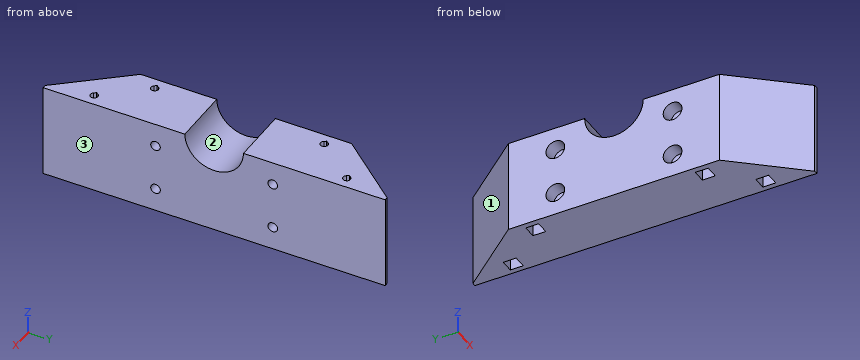
```python
from build123d import *

# Parameters (mm, degrees)
BOSS_EXTRUDE1_DEPTH   = 40
SKETCH2_R             = 2.05
CUT_EXTRUDE1_DEPTH    = 25.8
SKETCH2_4_R           = 4
SKETCH2_4_R_2         = 2.05
CUT_EXTRUDE2_DEPTH    = 6
CHAMFER1_SIZE2        = 2.5
CHAMFER1_SIZE         = 1.775056745
CHAMFER1_EDGE_2_SIZE2 = 2.5
CHAMFER1_EDGE_2_SIZE  = 1.775056745
SKETCH3_W             = 5.5
SKETCH3_H             = 5.5
CUT_EXTRUDE3_DEPTH    = 5


with BuildPart() as part:
    # Sketch1 → Boss-Extrude1 (new body)
    with BuildSketch(Plane(origin=(0, 0, 0), x_dir=(0, 1, 0), z_dir=(0, 0, 1))):
        Polygon((-45, 25), (45, 25), (74.76, 0.2), (-74.76, 0.2), align=None)
        with BuildLine():
            Line((-54.771952061, 6.432118468), (-53.854229763, 7.074714539))
            Line((-53.854229763, 7.074714539), (-52.936507465, 6.432118468))
            ThreePointArc((-52.936507465, 6.432118468), (-53.854229763, 3.521475197), (-54.771952061, 6.432118468))
        make_face(mode=Mode.SUBTRACT)
        with BuildLine():
            Line((-37.063492535, 21.189168074), (-36.145770237, 21.831764145))
            Line((-36.145770237, 21.831764145), (-35.228047939, 21.189168074))
            ThreePointArc((-35.228047939, 21.189168074), (-36.145770237, 18.278524803), (-37.063492535, 21.189168074))
        make_face(mode=Mode.SUBTRACT)
        with BuildLine():
            Line((35.228047939, 21.189168074), (36.145770237, 21.831764145))
            Line((36.145770237, 21.831764145), (37.063492535, 21.189168074))
            ThreePointArc((37.063492535, 21.189168074), (36.145770237, 18.278524803), (35.228047939, 21.189168074))
        make_face(mode=Mode.SUBTRACT)
        with BuildLine():
            Line((52.936507465, 6.432118468), (53.854229763, 7.074714539))
            Line((53.854229763, 7.074714539), (54.771952061, 6.432118468))
            ThreePointArc((54.771952061, 6.432118468), (53.854229763, 3.521475197), (52.936507465, 6.432118468))
        make_face(mode=Mode.SUBTRACT)
    extrude(amount=-BOSS_EXTRUDE1_DEPTH)

    # Sketch2 → Cut-Extrude1 (cut, through all)
    with BuildSketch(Plane(origin=(-25, 0, 0), x_dir=(0, -1, 0), z_dir=(-1, 0, 0))):
        with Locations((-25, -10)):
            Circle(SKETCH2_R)
        with Locations((-25, -30)):
            Circle(SKETCH2_R)
        with Locations((25, -30)):
            Circle(SKETCH2_R)
        with Locations((25, -10)):
            Circle(SKETCH2_R)
        with BuildLine():
            Line((12.5, 0), (-12.5, 0))
            ThreePointArc((-12.5, 0), (0, -12.5), (12.5, 0))
        make_face()
    extrude(amount=-CUT_EXTRUDE1_DEPTH, mode=Mode.SUBTRACT)

    # Sketch2_4 → Cut-Extrude2 (cut)
    with BuildSketch(Plane(origin=(-25, 0, 0), x_dir=(0, -1, 0), z_dir=(-1, 0, 0))):
        with Locations((-25, -10)):
            Circle(SKETCH2_4_R)
        with Locations((-25, -10)):
            Circle(SKETCH2_4_R_2, mode=Mode.SUBTRACT)
        with Locations((-25, -30)):
            Circle(SKETCH2_4_R)
        with Locations((-25, -30)):
            Circle(SKETCH2_4_R_2, mode=Mode.SUBTRACT)
        with Locations((25, -10)):
            Circle(SKETCH2_4_R)
        with Locations((25, -10)):
            Circle(SKETCH2_4_R_2, mode=Mode.SUBTRACT)
        with Locations((25, -30)):
            Circle(SKETCH2_4_R)
        with Locations((25, -30)):
            Circle(SKETCH2_4_R_2, mode=Mode.SUBTRACT)
        with BuildLine():
            Line((-12.5, 0), (12.5, 0))
            ThreePointArc((12.5, 0), (0, -12.5), (-12.5, 0))
        make_face()
    extrude(amount=-CUT_EXTRUDE2_DEPTH, mode=Mode.SUBTRACT)

    # Chamfer1
    chamfer1_edges = [part.edges().sort_by_distance(p)[0] for p in [
        (-0.2, 74.76, -20),
    ]]
    chamfer(chamfer1_edges, length=CHAMFER1_SIZE, length2=CHAMFER1_SIZE2)

    # Chamfer1 edge 2
    chamfer1_edge_2_edges = [part.edges().sort_by_distance(p)[0] for p in [
        (-0.2, -74.76, -20),
    ]]
    chamfer(chamfer1_edge_2_edges, length=CHAMFER1_EDGE_2_SIZE, length2=CHAMFER1_EDGE_2_SIZE2)

    # Sketch3 → Cut-Extrude3 (cut)
    with BuildSketch(Plane(origin=(0, 0, -40), x_dir=(1, 0, 0), z_dir=(0, 0, -1))):
        with Locations((-19.878524803, 36.145770237)):
            Rectangle(SKETCH3_W, SKETCH3_H)
        with Locations((-5.121475197, 53.854229763)):
            Rectangle(SKETCH3_W, SKETCH3_H)
        with Locations((-19.878524803, -36.145770237)):
            Rectangle(SKETCH3_W, SKETCH3_H)
        with Locations((-5.121475197, -53.854229763)):
            Rectangle(SKETCH3_W, SKETCH3_H)
    extrude(amount=-CUT_EXTRUDE3_DEPTH, mode=Mode.SUBTRACT)


solid = part.part
```
Can you work these out from the model? Positions are in its coordinate system, mm. Face numbers are marked on the shaded views. Give positions to 0.01 mm unless a question says otherwise; leave off trailing zeros. Write each loop counter-clockwise with the first axis right and the second up, starting at its lowest first coordinate (ties: lowest second). Pieces come first, ordered by that corner, then holes. Notation, with made-up numbers: (-25, 65) - (-13, 65) arc R13 ccw to (-13, 86) - close; hole circle Ø8 at (9.25, 54.5). An arc over 180 degrees is marked (long way). Write item = value, one per line. Start each with the question number.
1. For pin 1 (3 mm diameter, centred on x = -19.88, y = 36.15, fed in from +Z); pin 2 (2.5 mm diameter, centred on y = -52.5, z = -38, fed in from -X); pin 3 (5 mm diameter, centred on x = -18, z = -33, fed in from -Y); pin 4 (6.5 mm diameter, centred on y = 25, z = -10, fed in from -X), each with a flat end and sliding along its axis, tell me the tip position at first contact or that it passes through.
2. Please list where these lines run through material, in increasing order: line 1 (Z direction, x = -20.85, y = 25); line 2 (Y direction, x = -7, z = -11); line 3 (Y direction, x = -19.75, z = -25.5).
3. Imagine slicing it at B-B (z = -23.5). Please give me the cut outline in (x, y).
4. Thinking about a two-plate mould opening in Y: for the marked faces 1, 2 and 3, which applies, released by +Y, released by -Y, zero draft, split by the parting line, or undercut?
5. Imagine slicing it at C-C (y = -25). Please give me the cut outline in (x, z), and give its area (3 significant figures).
6. Imagine slicing it at A-A (z = -30). Count the separate pieces of the cut face and the enclosed holes in it, and give its area (3 significant figures).
7. Imagine slicing it at D-D (x = -10.75). Please give me the cut outline in (y, z).
Worked answers:
q1.pin_1 = through
q1.pin_2 = -19.79
q1.pin_3 = -56.4
q1.pin_4 = -19
q2.line_1 = -40 to -34, -26 to -14, -6 to 0
q2.line_2 = -66.6 to -53.96, -53.75 to -26.79, -23.21 to -5.94, 5.94 to 23.21, 26.79 to 53.75, 53.96 to 66.6
q2.line_3 = -51.3 to -37.74, -34.55 to 34.55, 37.74 to 51.3
q3.outline = (-25, -45) - (-1.8, -72.84) - (-0.2, -72.98) - (-0.2, 72.98) - (-1.8, 72.84) - (-25, 45) - close; hole (-21.83, -36.15) - (-21.19, -37.06) arc R1.6 ccw (long way) to (-21.19, -35.23) - close; hole (-21.83, 36.15) - (-21.19, 35.23) arc R1.6 ccw (long way) to (-21.19, 37.06) - close; hole (-7.07, -53.85) - (-6.43, -54.77) arc R1.6 ccw (long way) to (-6.43, -52.94) - close; hole (-7.07, 53.85) - (-6.43, 52.94) arc R1.6 ccw (long way) to (-6.43, 54.77) - close
q4.face_1 = released by +Y
q4.face_2 = undercut
q4.face_3 = zero draft
q5.outline = (-25, -40) - (-0.2, -40) - (-0.2, -32.05) - (-19, -32.05) - (-19, -34) - (-25, -34) - close; (-25, -26) - (-19, -26) - (-19, -27.95) - (-0.2, -27.95) - (-0.2, -12.05) - (-19, -12.05) - (-19, -14) - (-25, -14) - close; (-25, -6) - (-19, -6) - (-19, -7.95) - (-0.2, -7.95) - (-0.2, 0) - (-25, 0) - close
q5.area = 742 mm2
q6.separate_pieces = 3
q6.enclosed_holes = 4
q6.area = 2,680 mm2
q7.outline = (-62.1, -40) - (62.1, -40) - (62.1, 0) - (12.5, 0) arc R12.5 cw to (-12.5, 0) - (-62.1, 0) - close; hole circle Ø4.1 at (-25, -30); hole circle Ø4.1 at (-25, -10); hole circle Ø4.1 at (25, -30); hole circle Ø4.1 at (25, -10)
